Check sheet for the modelled part. Datum: model origin and axes. Units: mm. A direction names the side the tool comes from. Round coordinates to 2 decimals unless told otherwise and drop trailing zeros. Write each loop counter-clockwise with the first axis right and the second up, starting at its lowest first coordinate (ties: lowest second). Pieces come first, ordered by that corner, then holes. Notation, with made-up numbers: (34.25, 64.5) -> (77.25, 64.5) arc R21 ccw to (77.25, 68.5) -> close; hole circle Ø7 at (47.5, -15). An arc over 180 degrees is marked (long way). One line per item, written item: value.
from build123d import *

# Parameters (mm, degrees)
BOX011_W          = 7.8
BOX011_H          = 10
BOX011_DEPTH      = 2.8
FILLET003_R       = 0.8
BOX010_W          = 5.2
BOX010_H          = 50
BOX010_DEPTH      = 1.6
BOX008_W          = 57.2
BOX008_H          = 38.2
BOX008_DEPTH      = 1.6
CYLINDER012_R     = 16.7
CYLINDER012_DEPTH = 1.6
CYLINDER011_R     = 19.9
CYLINDER011_DEPTH = 17
BOX007_W          = 77.1
BOX007_H          = 39.8
BOX007_DEPTH      = 17
CYLINDER010_R     = 21.5
CYLINDER010_DEPTH = 17
BOX006_W          = 78.7
BOX006_H          = 43
BOX006_DEPTH      = 17
FILLET002_R       = 2.4
CHAMFER005_SIZE   = 0.8


with BuildPart() as usb:
    # Box011 → Box011 (new body)
    with BuildSketch(Plane(origin=(57.1, 45, 9.3), x_dir=(1, 0, 0), z_dir=(0, 0, 1))):
        with Locations((3.9, 5)):
            Rectangle(BOX011_W, BOX011_H)
    extrude(amount=BOX011_DEPTH)

    # Fillet003
    fillet003_edges = [usb.edges().sort_by_distance(p)[0] for p in [
        (57.1, 50, 12.1),
        (64.9, 50, 12.1),
    ]]
    fillet(fillet003_edges, radius=FILLET003_R)


with BuildPart() as obj1:
    # Box010 → Box010 (new body)
    with BuildSketch(Plane(origin=(37.9, 45, 13.8), x_dir=(1, 0, 0), z_dir=(0, 0, 1))):
        with Locations((2.6, 25)):
            Rectangle(BOX010_W, BOX010_H)
    extrude(amount=BOX010_DEPTH)


with BuildPart() as obj2:
    # Box008 → Box008 (new body)
    with BuildSketch(Plane(origin=(0, 50, 0), x_dir=(1, 0, 0), z_dir=(0, 0, 1))):
        with Locations((28.6, 19.1)):
            Rectangle(BOX008_W, BOX008_H)
    extrude(amount=BOX008_DEPTH)


with BuildPart() as zylinder012:
    # Cylinder012 → Cylinder012 (new body)
    with BuildSketch(Plane(origin=(76.2, 69.1, 0), x_dir=(1, 0, 0), z_dir=(0, 0, 1))):
        Circle(CYLINDER012_R)
    extrude(amount=CYLINDER012_DEPTH)


with BuildPart() as zylinder011:
    # Cylinder011 → Cylinder011 (new body)
    with BuildSketch(Plane(origin=(76.2, 69.1, 1.6), x_dir=(1, 0, 0), z_dir=(0, 0, 1))):
        Circle(CYLINDER011_R)
    extrude(amount=CYLINDER011_DEPTH)


with BuildPart() as fusion009:
    # Box007 → Box007 (new body)
    with BuildSketch(Plane(origin=(-0.8, 49.2, 1.6), x_dir=(1, 0, 0), z_dir=(0, 0, 1))):
        with Locations((38.55, 19.9)):
            Rectangle(BOX007_W, BOX007_H)
    extrude(amount=BOX007_DEPTH)

    # Fusion009: union Zylinder011
    add(zylinder011.part)


with BuildPart() as zylinder010:
    # Cylinder010 → Cylinder010 (new body)
    with BuildSketch(Plane(origin=(76.2, 69.1, 0), x_dir=(1, 0, 0), z_dir=(0, 0, 1))):
        Circle(CYLINDER010_R)
    extrude(amount=CYLINDER010_DEPTH)


with BuildPart() as top:
    # Box006 → Box006 (new body)
    with BuildSketch(Plane(origin=(-2.4, 47.6, 0), x_dir=(1, 0, 0), z_dir=(0, 0, 1))):
        with Locations((39.35, 21.5)):
            Rectangle(BOX006_W, BOX006_H)
    extrude(amount=BOX006_DEPTH)

    # Fusion008: union Zylinder010
    add(zylinder010.part)

    # Cut004: cut Fusion009
    add(fusion009.part, mode=Mode.SUBTRACT)

    # Fillet002
    fillet002_edges = [top.edges().sort_by_distance(p)[0] for p in [
        (-2.4, 47.6, 8.5),
        (-2.4, 90.6, 8.5),
    ]]
    fillet(fillet002_edges, radius=FILLET002_R)

    # Cut005: cut Zylinder012
    add(zylinder012.part, mode=Mode.SUBTRACT)

    # Cut006: cut obj2
    add(obj2.part, mode=Mode.SUBTRACT)

    # Chamfer005
    chamfer005_edges = [top.edges().sort_by_distance(p)[0] for p in [
        (57.2, 83.681153, 0),
        (28.6, 88.2, 0),
        (0, 69.1, 0),
        (28.6, 50, 0),
        (57.2, 54.518847, 0),
        (57.2, 69.1, 0),
    ]]
    chamfer(chamfer005_edges, length=CHAMFER005_SIZE)

    # Cut011: cut obj1
    add(obj1.part, mode=Mode.SUBTRACT)

    # Cut012: cut USB
    add(usb.part, mode=Mode.SUBTRACT)


solid = top.part
Item 1: Sectioned sample at B-B on y = 69.1. Enter the section's corners in (x, z).
Answer:
outline: (-2.4, 0) -> (-0.8, 0) -> (0, 0.8) -> (0, 1.6) -> (-0.8, 1.6) -> (-0.8, 17) -> (-2.4, 17) -> close; (57.2, 0.8) -> (58, 0) -> (59.5, 0) -> (59.5, 1.6) -> (57.2, 1.6) -> close; (92.9, 0) -> (97.7, 0) -> (97.7, 17) -> (96.1, 17) -> (96.1, 1.6) -> (92.9, 1.6) -> close
Item 2: Mould release check, pull along X, two halves, no side actions. Record for faces 3 (the flat face through (-0.8, 69, 9)), 4 (the flat face through (38, 90.6, 8)), 5 (the cylindrical face through (97.695, 68.629, 8.381)): pulls with the +X half, pulls with the -X half, needs draft (parallel to the pull), parting line crosses it, or undercut.
Answer:
face 3: undercut
face 4: needs draft
face 5: pulls with the +X half
Item 3: Sectioned sample at A-A on x = 16.5. Enter the section's corners in (y, z), and give its area (3 significant figures).
Answer:
outline: (47.6, 0) -> (49.2, 0) -> (50, 0.8) -> (50, 1.6) -> (49.2, 1.6) -> (49.2, 17) -> (47.6, 17) -> close; (88.2, 0.8) -> (89, 0) -> (90.6, 0) -> (90.6, 17) -> (89, 17) -> (89, 1.6) -> (88.2, 1.6) -> close
area: 56.3 mm^2
Item 4: Sectioned sample at D-D on y = 87. Enter the section's corners in (x, z), and give its area (3 significant figures).
Answer:
outline: (-2.4, 0) -> (-0.8, 0) -> (0, 0.8) -> (0, 1.6) -> (-0.8, 1.6) -> (-0.8, 17) -> (-2.4, 17) -> close; (57.2, 0.8) -> (58, 0) -> (88.11, 0) -> (88.11, 17) -> (84.89, 17) -> (84.89, 1.6) -> (57.2, 1.6) -> close
area: 127 mm^2
Item 5: Depth check by flat-ended pin: P1, Ø1.5, axis at y = 75, z = 2.5, coming from the +X side; P2, Ø0.8, axis at y = 49, z = 11, coming from the +X side; P3, Ø2, axis at y = 77.5, z = 9.5, coming from the +X side. Enter the tip coordinate at first touch or a pass-through.
Answer:
P1: stops at x = 97.07
P2: stops at x = 84.81
P3: stops at x = 96.39
Item 6: Thickness scan on line 1 (Y direction, x = 76.2, z = 0.8); line 2 (Y direction, x = 31.5, z = 8); line 3 (X direction, y = 77, z = 1.25). Record the ranges inside material, lowest first.
Answer:
line 1: y = 47.6 to 52.4, 85.8 to 90.6
line 2: y = 47.6 to 49.2, 89 to 90.6
line 3: x = -2.4 to 0, 57.2 to 61.49, 90.91 to 96.2
Item 7: Tool access check on faces 1 (the cylindrical face through (-1.678, 89.916, 8.619)), 2 (the flat face through (37, 89, 9)). Record the directions out of +Z, -Z, +X, -X, +Y, -Y that give a thin tool (end or side, any length) a straight path to the whole face; none if there is none.
Answer:
face 1: +Z, -Z, -X, +Y
face 2: +Z
